from build123d import *

# Parameters (mm, degrees)
F1_DEPTH      = 12.5
F3_W          = 2.5
F3_H          = 12.5
F4_DEPTH      = 9.464
F5_W          = 4.5
F5_H          = 14.5
F5_W_2        = 2.5
F5_H_2        = 12.5
F6_DEPTH      = 4
F6_DEPTH_BACK = 2
F7_R          = 0.5
F8_R          = 0.5


with BuildPart() as f1:
    # F0 (on Top) → F1 (new body)
    with BuildSketch(Plane.XY):
        Polygon((-13.8564064606, 0), (0, 0), (-3.4641016151, 6), align=None)
    extrude(amount=F1_DEPTH)

    # F3 (on offset) → F4 (join)
    with BuildSketch(Plane.YZ.offset(-3.4643)):
        with Locations((1.25, 6.25)):
            Rectangle(F3_W, F3_H)
    extrude(amount=F4_DEPTH)

    # F5 (on face) → F6 (join, two sides)
    with BuildSketch(Plane.YZ.offset(5.9997)) as f6_sk:
        with Locations((1.25, 6.25)):
            Rectangle(F5_W, F5_H)
        with Locations((1.25, 6.25)):
            Rectangle(F5_W_2, F5_H_2, mode=Mode.SUBTRACT)
    extrude(amount=F6_DEPTH)
    extrude(f6_sk.sketch, amount=-F6_DEPTH_BACK)

    # F7
    f7_edges = [f1.edges().sort_by_distance(p)[0] for p in [
        (-13.856406, 0, 6.25),
        (-3.464102, 6, 6.25),
    ]]
    fillet(f7_edges, radius=F7_R)

    # F8
    f8_edges = [f1.edges().sort_by_distance(p)[0] for p in [
        (3.9997, 1.25, 0),
        (3.9997, 0, 6.25),
        (3.9997, 2.5, 6.25),
        (3.9997, 1.25, 12.5),
        (6.9997, -1, 13.5),
        (6.9997, 3.5, 13.5),
        (6.9997, 3.5, -1),
        (6.9997, -1, -1),
    ]]
    fillet(f8_edges, radius=F8_R)


solid = f1.part
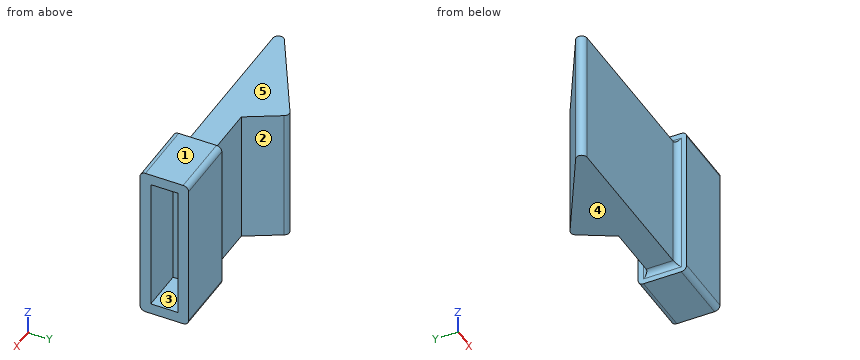
Could you check a few things on this model? Use its own coordinates, in mm. Face numbers are marked on the shaded views. A direction names the side the tool comes from. Coordinates: 2 decimals unless noted, no trailing zeros. Write each loop counter-clockwise with the first axis right and the second up, starting at its lowest first coordinate (ties: lowest second). Pieces come first, ordered by that corner, then holes. Notation, with made-up numbers: (42.5, 55.25) - (99.5, 55.25) arc R25 cw to (99.5, 80.25) - close; hole circle Ø5 at (80, 82.25). An arc over 180 degrees is marked (long way). Write item = value, one per line.
1) Please list where these lines run through material, in increasing order: line 1 (Y direction, x = 6.5, z = 8.5); line 2 (Z direction, x = -7.5, y = 3.5); line 3 (Y direction, x = 8.5, z = 12.75). Write a range as [from, to].
Result set:
line_1 = [-1, 0], [2.5, 3.5]
line_2 = [0, 12.5]
line_3 = [-1, 3.5]
2) For the marked faces 3, 4 and 5, which set-ups out of +Z, -Z, +X, -X, +Y, -Y let a thin tool reach every point of the face, with its end or its side?
Result set:
face_3 = +X
face_4 = -Z, -X, +Y, -Y
face_5 = +Z, -X, +Y, -Y
3) Suppose I cut it at D-D on y = 4.25. Please give me the cut outline in (x, z).
Result set:
outline = (-6.5, 0) - (-2.45, 0) - (-2.45, 12.5) - (-6.5, 12.5) - close
4) Suppose I cut it at B-B on z = 5. Please give me the cut outline in (x, y), plus the area to 3 significant figures.
Result set:
outline = (-12.24, 0.93) arc R0.5 ccw to (-11.99, 0) - (3.5, 0) arc R0.5 cw to (4, -0.5) - (4, -1) - (10, -1) - (10, 0) - (6, 0) - (6, 2.5) - (10, 2.5) - (10, 3.5) - (4, 3.5) - (4, 3) arc R0.5 cw to (3.5, 2.5) - (-1.44, 2.5) - (-3.21, 5.57) arc R0.5 ccw to (-3.9, 5.75) - close
area = 69.8 mm2
5) Will these pins go through, and if not, where does the flat tip stop? pin 1 Ø1 at (x, z) = (-1, 9.5) entering from +Y; pin 2 Ø1 at (x, y) = (-4.5, 3) entering from -Z; pin 3 Ø5 at (x, z) = (8.5, 3.5) entering from +Y.
Result set:
pin_1 = 2.6
pin_2 = 0
pin_3 = 3.5
6) We'd pull the mould along X, two halves only. Please class the marked faces 1 and 2: +X half, -X half, draft (parallel to the pull), parting line (faces both ways), or undercut.
Result set:
face_1 = draft
face_2 = undercut
7) Suppose I cut it at A-A on x = 8.5. Please give me the cut outline in (y, z).
Result set:
outline = (-1, -0.5) arc R0.5 ccw to (-0.5, -1) - (3, -1) arc R0.5 ccw to (3.5, -0.5) - (3.5, 13) arc R0.5 ccw to (3, 13.5) - (-0.5, 13.5) arc R0.5 ccw to (-1, 13) - close; hole (0, 0) - (2.5, 0) - (2.5, 12.5) - (0, 12.5) - close
8) Suppose I cut it at C-C on x = 5.5. Please give me the cut outline in (y, z), plus the area to 3 significant figures.
Result set:
outline = (-1, -0.5) arc R0.5 ccw to (-0.5, -1) - (3, -1) arc R0.5 ccw to (3.5, -0.5) - (3.5, 13) arc R0.5 ccw to (3, 13.5) - (-0.5, 13.5) arc R0.5 ccw to (-1, 13) - close
area = 65.0 mm2
